from build123d import *

# Parameters (mm, degrees)
F0_R     = 50.2290121712
F0_R_2   = 39.7205191913
F1_DEPTH = 60.452
F2_R     = 50.1012725797
F3_DEPTH = 15.24
F4_R     = 2.4528409794


# Not quite as in the source:
# - a feature names something its author has since deleted; it is built from what else it names


with BuildPart() as f1:
    # F0 (on Top) → F1 (new body)
    with BuildSketch(Plane.XY):
        Circle(F0_R)
        Circle(F0_R_2, mode=Mode.SUBTRACT)
    extrude(amount=F1_DEPTH)

    # F2 (on face) → F3 (join)
    with BuildSketch(Plane(origin=(0, 0, 0), x_dir=(1, 0, 0), z_dir=(0, 0, -1))):
        Circle(F2_R)
    extrude(amount=F3_DEPTH)

    # F4
    f4_edges = [f1.edges().sort_by_distance(p)[0] for p in [
        (-50.229012, 0, 60.452),
        (-39.720519, 0, 60.452),
    ]]
    fillet(f4_edges, radius=F4_R)


solid = f1.part
Could you check a few things on this model? Use its own coordinates, in mm. Give positions to 0.01 mm unless a question says otherwise; leave off trailing zeros. Loops run counter-clockwise (first coordinate to the right, second up) from the corner with the lowest first, then second, coordinate; pieces in that order, holes last. Notation, with made-up numbers: M -10.5,-21.75 L 7.5,-21.75 A13 cw 7.5,-2.75 Z; hole C 65,78 d9. An arc over 180 degrees is marked long. Answer as a JSON object with one key per item and string values.
Q1. Suppose I cut it at C-C, the plane z = 7. List the corners of the cut face in (x, y) for me, plus the area to 3 significant figures.
Values found:
{"outline": "C 0,0 d100.46; hole C 0,0 d79.44", "area": "2,970 mm²"}
Q2. If we mould it in two halves opening along Y, with no side actions, what happens to faces 1 (the cylindrical face through (21.354, 33.492, 28.594)), 2 (the flat face through (-1, -1, 0)), 3 (the cylindrical face through (-10.9, 48.9, -7.5)), 4 (the flat face through (3.3, -42.2, 60.452))? For each: pulls with the +Y half, pulls with the -Y half, needs draft (parallel to the pull), parting line crosses it, or undercut.
Values found:
{"face 1": "undercut", "face 2": "undercut", "face 3": "parting line crosses it", "face 4": "needs draft"}
Q3. For P1, Ø2, axis at y = 7, z = 15.5, coming from the -X side; P2, Ø5, axis at y = 13, z = 35, coming from the +X side; P3, Ø1.5, axis at y = 19.5, z = 29, coming from the -X side; P4, Ø12, axis at x = -35.5, y = 14, coming from the +Z side, each with a flat end and sliding along its axis, tell me the tip position at first contact or that it passes through.
Values found:
{"P1": "stops at x = -49.87", "P2": "stops at x = 49.12", "P3": "stops at x = -46.6", "P4": "stops at z = 60.45"}
Q4. Suppose I cut it at A-A, the plane x = 0. List the corners of the cut face in (y, z) for me, plus the area to 3 significant figures.
Values found:
{"outline": "M -50.23,0 L -50.1,0 L -50.1,-15.24 L 50.1,-15.24 L 50.1,0 L 50.23,0 L 50.23,58 A2.45 ccw 47.78,60.45 L 42.17,60.45 A2.45 ccw 39.72,58 L 39.72,0 L -39.72,0 L -39.72,58 A2.45 ccw -42.17,60.45 L -47.78,60.45 A2.45 ccw -50.23,58 Z", "area": "2,790 mm²"}
Q5. If I drill on probe 1 along Y at (x, z) = (0, 28.5); probe 2 along Z at (x, y) = (-12, 27.5); probe 3 along Z at (x, y) = (-37.5, -18.5), over which ranges is the centre line in solid material (lowest first)? Write a range as [from, to].
Values found:
{"probe 1": "y = [-50.23, -39.72], [39.72, 50.23]", "probe 2": "z = [-15.24, 0]", "probe 3": "z = [-15.24, 60.43]"}
